Geometry check sheet. Reference: the model listing, model coordinates, mm. Face numbers are marked on the shaded views. A direction names the side the tool comes from. Give positions to 0.01 mm unless a question says otherwise; leave off trailing zeros. Order: outer loops, then holes, each group sorted by start corner. A loop starts at its lowest first (then second) coordinate and runs counter-clockwise, first axis right, second up. Notation, with made-up numbers: M 58.25,-13 L 62.25,-13 A34 cw 62.25,26 Z; hole C 36,17.25 d8. An arc over 180 degrees is marked long. One line per question, with ' | ' between items. Start each with the question number.
from build123d import *

# Parameters (mm, degrees)
SKETCH_1_R               = 52.5
EXTRUDE_1_DEPTH          = 60
SKETCH_2_R               = 37.5
EXTRUDE_2_DEPTH          = 40
SKETCH_3_R               = 42.5
CUT_EXTRUDE_1_DEPTH      = 40
SKETCH_4_R               = 22.5
CUT_EXTRUDE_2_DEPTH      = 125.549187071
CHAMFER_1_SIZE           = 1
CUT_EXTRUDE_3_DEPTH      = 125.549187071
CUT_EXTRUDE_3_DEPTH_BACK = 125.549187071
SKETCH_5_R               = 5
CHAMFER_2_SIZE           = 5


with BuildPart() as part:
    # Эскиз1 → Бобышка-Вытянуть1 (new body)
    with BuildSketch(Plane.XY):
        Circle(SKETCH_1_R)
    extrude(amount=EXTRUDE_1_DEPTH)

    # Эскиз2 → Бобышка-Вытянуть2 (add)
    with BuildSketch(Plane.XY.offset(60)):
        Circle(SKETCH_2_R)
    extrude(amount=EXTRUDE_2_DEPTH)

    # Эскиз3 → Вырез-Вытянуть1 (cut)
    with BuildSketch(Plane(origin=(0, 0, 0), x_dir=(-1, 0, 0), z_dir=(0, 0, -1))):
        Circle(SKETCH_3_R)
    extrude(amount=-CUT_EXTRUDE_1_DEPTH, mode=Mode.SUBTRACT)

    # Эскиз4 → Вырез-Вытянуть2 (cut, through all)
    with BuildSketch(Plane.XY.offset(100)):
        Circle(SKETCH_4_R)
    extrude(amount=-CUT_EXTRUDE_2_DEPTH, mode=Mode.SUBTRACT)

    # Фаска1
    chamfer_1_edges = [part.edges().sort_by_distance(p)[0] for p in [
        (42.5, 0, 0),
        (-52.5, 0, 0),
    ]]
    chamfer(chamfer_1_edges, length=CHAMFER_1_SIZE)

    # Эскиз5 → Вырез-Вытянуть3 (cut, two sides: drawn at the far end of the back side and taken through both)
    with BuildSketch(Plane(origin=(0, 0, 0), x_dir=(0, 0, -1), z_dir=(1, 0, 0)).offset(-CUT_EXTRUDE_3_DEPTH_BACK)):
        with Locations((-80, 0)):
            Circle(SKETCH_5_R)
    extrude(amount=CUT_EXTRUDE_3_DEPTH + CUT_EXTRUDE_3_DEPTH_BACK, mode=Mode.SUBTRACT)

    # Фаска2
    chamfer_2_edges = [part.edges().sort_by_distance(p)[0] for p in [
        (-22.5, 0, 100),
        (-37.5, 0, 100),
    ]]
    chamfer(chamfer_2_edges, length=CHAMFER_2_SIZE)


solid = part.part
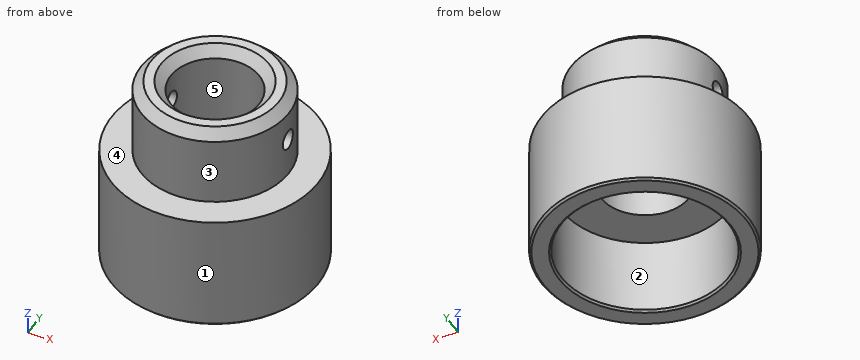
Item 1: Material ranges on line 1 along X through (y, z) = (0, 66); line 2 along Y through (x, z) = (0, 20.5); line 3 along Z through (x, y) = (28, 0), recorded low to high.
Item 2: Cross-section at C-C, the plane z = 67.5. Record the cut outline in (x, y).
Item 3: Cross-section at B-B, the plane y = 0. State how many separate pieces and enclosed holes the cut face has, plus the area to 3 significant figures.
Item 4: Cross-section at D-D, the plane z = 80. Record the cut outline in (x, y), plus the area to 3 significant figures.
Item 5: Mould release check, pull along Y, two halves, no side actions. Record for the marked faces 3, 4 and 5: released by +Y, released by -Y, zero draft, split by the parting line, or undercut.
Item 6: Cross-section at A-A, the plane x = 0. Record the cut outline in (y, z), plus the area to 3 significant figures.
Item 7: Depth check by flat-ended pin: pin 1 (10 mm diameter, centred on x = -6, z = 24, fed in from -Y); pin 2 (13 mm diameter, centred on y = 0, z = 80, fed in from +X); pin 3 (3 mm diameter, centred on x = -10.5, z = 68.5, fed in from +Y). Enter the tip coordinate at first touch or a pass-through.
Item 8: Set-up check for the marked faces 1 and 2: record each of +Z, -Z, +X, -X, +Y, -Y from which the full face is reachable in a straight line by a thin tool's end or side.
Outcome:
1) line 1: x = -37.5 to -22.5, 22.5 to 37.5 | line 2: y = -52.5 to -42.5, 42.5 to 52.5 | line 3: z = 40 to 75, 85 to 100
2) outline: C 0,0 d75; hole C 0,0 d45
3) separate pieces: 4 | enclosed holes: 0 | area: 2,850 mm²
4) outline: M -37.17,-5 A37.5 ccw 37.17,-5 L 21.94,-5 A22.5 cw -21.94,-5 Z; M -37.17,5 L -21.94,5 A22.5 cw 21.94,5 L 37.17,5 A37.5 ccw Z | area: 2,530 mm²
5) face 3: split by the parting line | face 4: zero draft | face 5: undercut
6) outline: M -52.5,1 L -51.5,0 L -43.5,0 L -42.5,1 L -42.5,40 L -22.5,40 L -22.5,95 L -27.5,100 L -32.5,100 L -37.5,95 L -37.5,60 L -52.5,60 Z; M 22.5,40 L 42.5,40 L 42.5,1 L 43.5,0 L 51.5,0 L 52.5,1 L 52.5,60 L 37.5,60 L 37.5,95 L 32.5,100 L 27.5,100 L 22.5,95 Z | area: 3,150 mm²
7) pin 1: stops at y = -52.49 | pin 2: stops at x = 37.5 | pin 3: stops at y = 36.4
8) face 1: +Z, -Z | face 2: -Z
